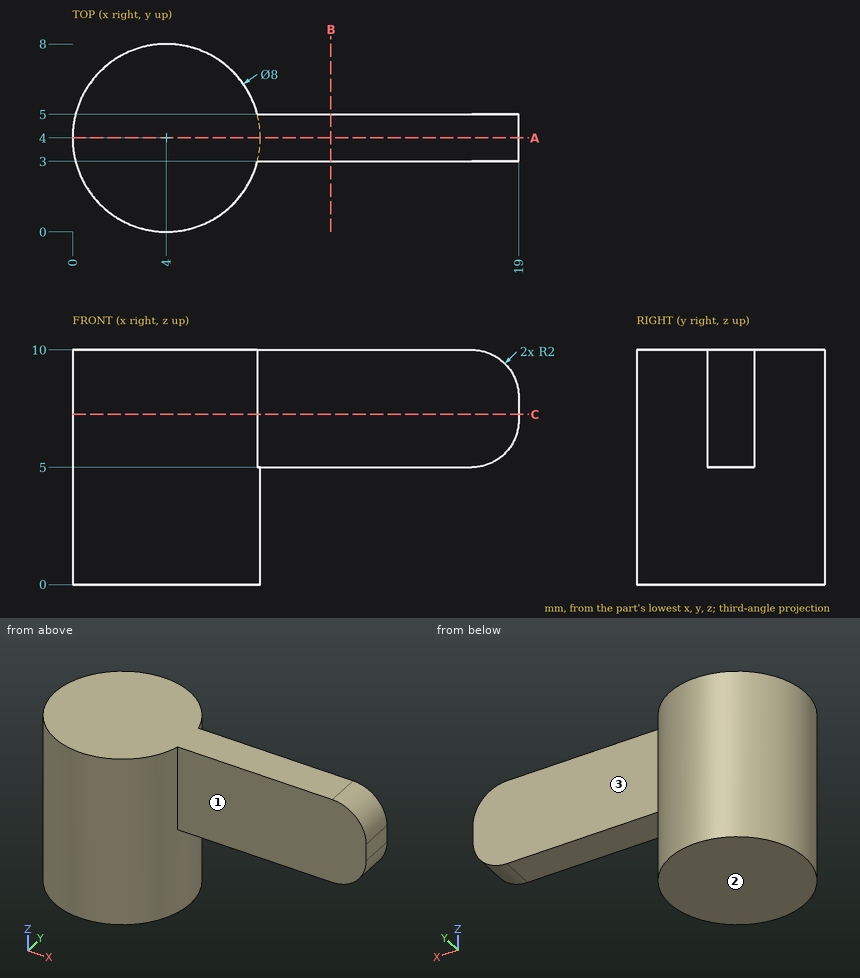
Here's the drawing with two shaded views (mm, measured from the low corner). I have some questions. A direction names the side the tool comes from. Give positions to 0.01 mm unless a question says otherwise; leave off trailing zeros. Order: outer loops, then holes, each group sorted by start corner. A loop starts at its lowest first (then second) coordinate and runs counter-clockwise, first axis right, second up. Notation, with made-up numbers: (59.25, 10.5) -> (72.25, 10.5) arc R21 cw to (72.25, 22.5) -> close; hole circle Ø8 at (-24.5, 72). An arc over 180 degrees is marked (long way). Use a Markdown table: item, result. Add a question column.
Item 1: Imagine slicing it at C-C on z = 7.25. Please give me the cut outline in (x, y), plus the area to 3 significant figures.
Item 2: For the marked faces 1, 2 and 3, which set-ups out of +Z, -Z, +X, -X, +Y, -Y let a thin tool reach every point of the face, with its end or its side?
Item 3: Will these pins go through, and if not, where does the flat tip stop? pin 1 (5.5 mm diameter, centred on x = 16, z = 7.5, fed in from -Y); pin 2 (3 mm diameter, centred on y = 3, z = 1.5, fed in from -X); pin 3 (1.6 mm diameter, centred on x = 14, y = 3.5, fed in from -Z); pin 4 (4 mm diameter, centred on x = 13, z = 7, fed in from +Y).
Item 4: Imagine slicing it at A-A on y = 4. Please give me the cut outline in (x, z).
Item 5: Imagine slicing it at B-B on x = 11. Please give me the cut outline in (y, z).
Item 6: I need wall thicknesses on line 1 (Z direction, x = 17.25, y = 3.25); line 2 (X direction, y = 7, z = 4); line 3 (X direction, y = 2.5, z = 6.75). Which ranges of each line are inside material? Lowest first, please.
Data:
| question | item | result |
|---|---|---|
| 1 | outline | (7.87, 3) -> (19, 3) -> (19, 5) -> (7.87, 5) arc R4 ccw (long way) to start |
| 1 | area | 72.3 mm² |
| 2 | face 1 | +Z, -Z, +X, -Y |
| 2 | face 2 | -Z, +X, -X, +Y, -Y |
| 2 | face 3 | +Z, -Z, +X, +Y |
| 3 | pin 1 | stops at y = 3 |
| 3 | pin 2 | stops at x = 0 |
| 3 | pin 3 | stops at z = 5 |
| 3 | pin 4 | stops at y = 5 |
| 4 | outline | (0, 0) -> (8, 0) -> (8, 5) -> (17, 5) arc R2 ccw to (19, 7) -> (19, 8) arc R2 ccw to (17, 10) -> (0, 10) -> close |
| 5 | outline | (3, 5) -> (5, 5) -> (5, 10) -> (3, 10) -> close |
| 6 | line 1 | z = 5.02 to 9.98 |
| 6 | line 2 | x = 1.35 to 6.65 |
| 6 | line 3 | x = 0.29 to 7.71 |
